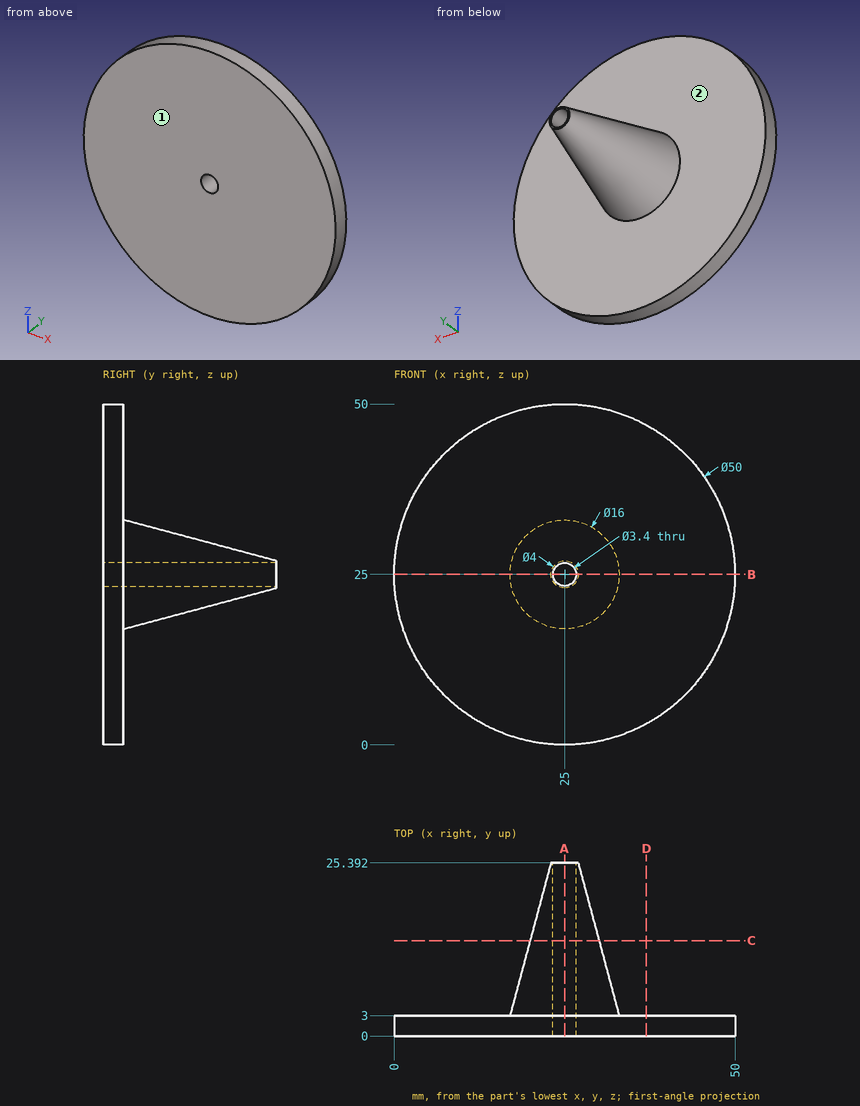
Could you check a few things on this drawing? It's one solid part, dimensions in mm from its lowest x, y, z. A direction names the side the tool comes from. Coordinates: 2 decimals unless noted, no trailing zeros. Write each loop counter-clockwise with the first axis right and the second up, starting at its lowest first coordinate (ties: lowest second). Pieces come first, ordered by that corner, then holes. Notation, with made-up numbers: M 39.5,9.25 L 93.5,9.25 A19 ccw 93.5,21.25 Z; hole C 28,73.5 d9. An arc over 180 degrees is marked long. One line per question, with ' | ' between items.
1) For the marked faces 1 and 2, which set-ups out of +Z, -Z, +X, -X, +Y, -Y let a thin tool reach every point of the face, with its end or its side?
Checks:
face 1: +Z, -Z, +X, -X, -Y | face 2: +Y
2) Imagine slicing it at C-C, the plane y = 14. Write out the boundary of the cut face in (x, z) (1 decimal).
Checks:
outline: C 25,25 d10.1; hole C 25,25 d3.4
3) Imagine slicing it at D-D, the plane x = 37. Write out the boundary of the cut face in (y, z), and give its area (3 significant figures).
Checks:
outline: M 0,3.07 L 3,3.07 L 3,46.93 L 0,46.93 Z | area: 132 mm²
4) Imagine slicing it at B-B, the plane z = 25. Write out the boundary of the cut face in (x, y).
Checks:
outline: M 0,0 L 23.3,0 L 23.3,25.39 L 23,25.39 L 17,3 L 0,3 Z; M 26.7,0 L 50,0 L 50,3 L 33,3 L 27,25.39 L 26.7,25.39 Z
5) For pin 1 Ø5 at (y, z) = (5, 37.5) entering from -X; pin 2 Ø1.5 at (y, z) = (3, 31.5) entering from -X; pin 3 Ø1.5 at (y, z) = (5.5, 30.5) entering from +X (1 decimal), each with a flat end and sliding along its axis, tell me the tip position at first contact or that it passes through.
Checks:
pin 1: x = 2.55 | pin 2: x = 0.67 | pin 3: x = 30.6
6) I need wall thicknesses on probe 1 along Y at (x, z) = (35.5, 25.5); probe 2 along X at (y, z) = (9.25, 25.5) (1 decimal); probe 3 along X at (y, z) = (18.25, 25). Which ranges of each line are inside material? Lowest first, please. Write a range as [from, to].
Checks:
probe 1: [0, 3] | probe 2: [18.7, 23.4], [26.6, 31.3] | probe 3: [21.09, 23.3], [26.7, 28.91]
7) Imagine slicing it at A-A, the plane x = 25. Write out the boundary of the cut face in (y, z).
Checks:
outline: M 0,0 L 3,0 L 3,17 L 25.39,23 L 25.39,23.3 L 0,23.3 Z; M 0,26.7 L 25.39,26.7 L 25.39,27 L 3,33 L 3,50 L 0,50 Z
